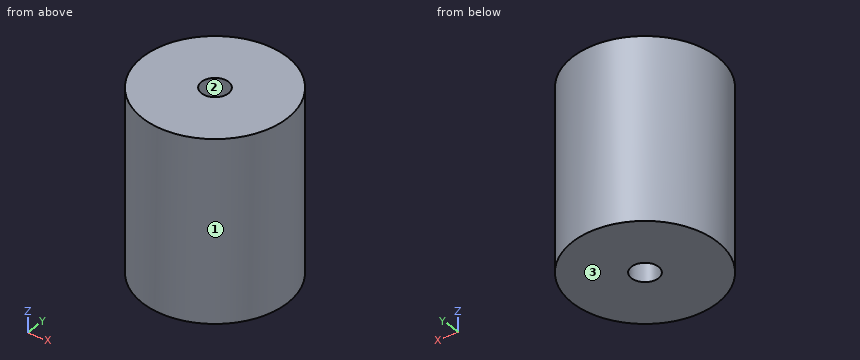
from build123d import *

# Parameters (mm, degrees)
F0_R     = 50.8
F1_DEPTH = 63.5
F2_D     = 19.05
F3_D     = 19.05


with BuildPart() as f1:
    # F0 (on Top) → F1 (new body, symmetric)
    with BuildSketch(Plane.XY):
        Circle(F0_R)
    extrude(amount=F1_DEPTH, both=True)

    # F2 (through all)
    with Locations(Plane.XY):
        with Locations((0, 0)):
            Hole(F2_D / 2)

    # F3 (through all)
    with Locations(Plane(origin=(0, 0, 0), x_dir=(1, 0, 0), z_dir=(0, 0, -1))):
        with Locations((0, 0)):
            Hole(F3_D / 2)


solid = f1.part
Geometry: final body of the model. Coordinates: model frame, mm. Face numbers are marked on the shaded views. Coordinates: 2 decimals unless noted, no trailing zeros. Loops run counter-clockwise (first coordinate to the right, second up) from the corner with the lowest first, then second, coordinate; pieces in that order, holes last. Notation, with made-up numbers: M 14.5,19 L 31.5,19 A33 ccw 31.5,53 Z; hole C -34,40 d4. An arc over 180 degrees is marked long. One line per item, written item: value. Start each with the question number.
1) Cut plane C-C (z = 47.5). Return loops of the section in (x, y) (3 decimals), then the cut area to 3 significant figures.
2) Cut plane A-A (y = 0). Return loops of the section in (x, z) (3 decimals).
3) Material intervals for L1, parallel to Y at x = 0, z = 14 (3 decimals); L2, parallel to X at y = -0.5, z = -53; L3, parallel to X at y = -6.5, z = 57, sorted ascending. Write a range as from..to.
4) Cut plane D-D (y = 20.5). Return loops of the section in (x, z).
5) Draft query along Y for the marked faces 1, 2 and 3. Return one class per face: released by +Y, released by -Y, zero draft, split by the parting line, or undercut.
6) Pin query (flat end, axial travel): P1, Ø6, axis at x = -38.5, z = 45, coming from the +Y side; P2, Ø1.5, axis at x = -34.5, z = 10, coming from the -Y side; P3, Ø2, axis at x = -27.5, z = 46.5, coming from the -Y side. Return the tip coordinate at first contact, or that it passes through.
Evaluation:
1. outline: C 0,0 d101.6; hole C 0,0 d19.05
1. area: 7,820 mm^2
2. outline: M -50.8,-63.5 L -9.525,-63.5 L -9.525,63.5 L -50.8,63.5 Z; M 9.525,-63.5 L 50.8,-63.5 L 50.8,63.5 L 9.525,63.5 Z
3. L1: -50.8..-9.525, 9.525..50.8
3. L2: -50.8..-9.51, 9.51..50.8
3. L3: -50.38..-6.96, 6.96..50.38
4. outline: M -46.48,-63.5 L 46.48,-63.5 L 46.48,63.5 L -46.48,63.5 Z
5. face 1: split by the parting line
5. face 2: undercut
5. face 3: zero draft
6. P1: y = 36.34
6. P2: y = -37.97
6. P3: y = -43.34
